from build123d import *

# Parameters (mm, degrees)
SKETCH_1_W          = 30
SKETCH_1_H          = 50
EXTRUDE_1_DEPTH     = 500
SKETCH_2_R          = 10
CUT_EXTRUDE_1_DEPTH = 503.717614571
SKETCH_3_R          = 10
CUT_EXTRUDE_2_DEPTH = 502.522681441


with BuildPart() as part:
    # Эскиз1 → Бобышка-Вытянуть1 (new body)
    with BuildSketch(Plane.XY):
        Rectangle(SKETCH_1_W, SKETCH_1_H)
    extrude(amount=EXTRUDE_1_DEPTH)

    # Эскиз2 → Вырез-Вытянуть1 (cut, through all)
    with BuildSketch(Plane(origin=(0, 25, 0), x_dir=(1, 0, 0), z_dir=(0, 1, 0))):
        with Locations(Location((0, -90, 0), (0, 0, 270))):
            Circle(SKETCH_2_R)
        with Locations(Location((0, -410, 0), (0, 0, 90))):
            Circle(SKETCH_2_R)
    extrude(amount=-CUT_EXTRUDE_1_DEPTH, mode=Mode.SUBTRACT)

    # Эскиз3 → Вырез-Вытянуть2 (cut, through all)
    with BuildSketch(Plane.ZY.offset(15)):
        with Locations(Location((250, 0, 0), (0, 0, 270))):
            Circle(SKETCH_3_R)
    extrude(amount=-CUT_EXTRUDE_2_DEPTH, mode=Mode.SUBTRACT)


solid = part.part
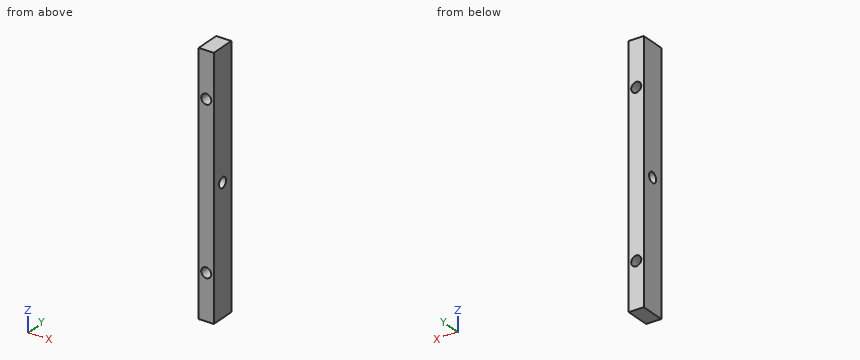
Input: part model. Units: mm. Frame: model coordinates. Coordinates: 2 decimals unless noted, no trailing zeros. Order: outer loops, then holes, each group sorted by start corner. A loop starts at its lowest first (then second) coordinate and runs counter-clockwise, first axis right, second up. Notation, with made-up numbers: M 66,-0.75 L 84,-0.75 A20 ccw 84,9.25 Z; hole C 25,55 d9. An arc over 180 degrees is marked long. Answer in a Markdown table with one row per item.
(1) Section query B-B, the plane z = 90. Output: boundary loops of the cut face in (x, y).
Numbers:
| item | result |
|---|---|
| outline | M -15,-25 L -10,-25 L -10,25 L -15,25 Z; M 10,-25 L 15,-25 L 15,25 L 10,25 Z |
(2) Section query D-D, the plane y = -20.5. Output: boundary loops of the cut face in (x, z), plus the area to 3 significant figures.
Numbers:
| item | result |
|---|---|
| outline | M -15,0 L 15,0 L 15,500 L -15,500 Z; hole C 0,90 d20; hole C 0,410 d20 |
| area | 14,400 mm^2 |
(3) Contact query for a flat-ended pin moving along its axis: pin 1 Ø16 at (x, z) = (0, 410) entering from -Y (3 decimals). Output: stop coordinate, or through.
Numbers:
| item | result |
|---|---|
| pin 1 | passes through |
(4) Section query A-A, the plane x = 0. Output: boundary loops of the cut face in (y, z), plus the area to 3 significant figures.
Numbers:
| item | result |
|---|---|
| outline | M -25,0 L 25,0 L 25,80 L -25,80 Z; M -25,100 L 25,100 L 25,400 L -25,400 Z; M -25,420 L 25,420 L 25,500 L -25,500 Z; hole C 0,250 d20 |
| area | 22,700 mm^2 |
(5) Material intervals for line 1 (Z direction, x = 0.5, y = 1); line 2 (Z direction, x = 0.5, y = 0); line 3 (X direction, y = 3, z = 410), sorted ascending. Write a range as [from, to].
Numbers:
| item | result |
|---|---|
| line 1 | z = [0, 80.01], [99.99, 240.05], [259.95, 400.01], [419.99, 500] |
| line 2 | z = [0, 80.01], [99.99, 240], [260, 400.01], [419.99, 500] |
| line 3 | x = [-15, -10], [10, 15] |
(6) Section query C-C, the plane y = 0. Output: boundary loops of the cut face in (x, z).
Numbers:
| item | result |
|---|---|
| outline | M -15,0 L 15,0 L 15,240 L -15,240 Z; M -15,260 L 15,260 L 15,500 L -15,500 Z; hole C 0,90 d20; hole C 0,410 d20 |
